Can you work these out from the model? Positions are in its coordinate system, mm. A direction names the side the tool comes from. Give positions to 0.01 mm unless a question says otherwise; leave off trailing zeros. Loops run counter-clockwise (first coordinate to the right, second up) from the corner with the lowest first, then second, coordinate; pieces in that order, holes last. Notation, with made-up numbers: M 85.5,53.5 L 108.5,53.5 A26 ccw 108.5,78.5 Z; hole C 88.5,56 d1. An arc over 180 degrees is marked long. Answer as a JSON object with one key per item and string values.
```python
from build123d import *

# Parameters (mm, degrees)
BOSS_EXTRUDE1_DEPTH = 60
SKETCH2_W           = 45
SKETCH2_H           = 21
CUT_EXTRUDE1_DEPTH  = 6
SKETCH3_W           = 6
SKETCH3_H           = 6
BOSS_EXTRUDE2_DEPTH = 18


with BuildPart() as part:
    # Sketch1 → Boss-Extrude1 (new body)
    with BuildSketch(Plane.XY):
        Polygon((50, 0), (-50, 0), (-69.206794991, 50), (-63.605822035, 52.151534787), (-45.877360691, 6), (45.877360691, 6), (63.605822035, 52.151534787), (69.206794991, 50), align=None)
    extrude(amount=BOSS_EXTRUDE1_DEPTH)

    # Sketch2 → Cut-Extrude1 (cut)
    with BuildSketch(Plane.XZ):
        with Locations((0, 18.669109879)):
            Rectangle(SKETCH2_W, SKETCH2_H)
    extrude(amount=-CUT_EXTRUDE1_DEPTH, mode=Mode.SUBTRACT)

    # Sketch3 → Boss-Extrude2 (add)
    with BuildSketch(Plane.XZ):
        with Locations((-19.5, 40.5)):
            Rectangle(SKETCH3_W, SKETCH3_H)
        with Locations((19.5, 40.5)):
            Rectangle(SKETCH3_W, SKETCH3_H)
    extrude(amount=BOSS_EXTRUDE2_DEPTH)


solid = part.part
```
1) For faces 1 (the flat face through (-16.5, -9, 40)), 2 (the flat face through (-20, -9, 43.5)), 3 (the flat face through (0, 3, 8.169)), 4 (the flat face through (-1, 6, 30)), which set-ups out of +Z, -Z, +X, -X, +Y, -Y let a thin tool reach every point of the face, with its end or its side?
Answer list:
{"face 1": "+Z, -Z, -Y", "face 2": "+Z, +X, -X, -Y", "face 3": "+Y, -Y", "face 4": "+Z, -Z, +Y"}
2) Suppose I cut it at D-D, the plane z = 54.5. Write out the boundary of the cut face in (x, y), and give its area (3 significant figures).
Answer list:
{"outline": "M -69.21,50 L -50,0 L 50,0 L 69.21,50 L 63.61,52.15 L 45.88,6 L -45.88,6 L -63.61,52.15 Z", "area": "1,190 mm^2"}
3) If we mould it in two halves opening along X, with no side actions, what happens to faces 5 (the flat face through (66.37, 51.09, 29.58)), 6 (the flat face through (0, 3, 29.169)), 7 (the flat face through (19, -9, 37.5))? For each: +X half, -X half, draft (parallel to the pull), parting line (faces both ways), or undercut.
Answer list:
{"face 5": "+X half", "face 6": "undercut", "face 7": "draft"}
4) Suppose I cut it at A-A, the plane x = 14. Write out the boundary of the cut face in (y, z), and give its area (3 significant figures).
Answer list:
{"outline": "M 0,0 L 6,0 L 6,8.17 L 0,8.17 Z; M 0,29.17 L 6,29.17 L 6,60 L 0,60 Z", "area": "234 mm^2"}
5) Suppose I cut it at B-B, the plane z = 24.5. Write out the boundary of the cut face in (x, y).
Answer list:
{"outline": "M -69.21,50 L -50,0 L -22.5,0 L -22.5,6 L -45.88,6 L -63.61,52.15 Z; M 22.5,0 L 50,0 L 69.21,50 L 63.61,52.15 L 45.88,6 L 22.5,6 Z"}
6) Will these pins go through, and if not, where does the flat tip stop? pin 1 Ø3 at (x, y) = (-6, 4) entering from -Z; pin 2 Ø6.5 at (x, y) = (-21, -5.5) entering from -Z; pin 3 Ø18 at (x, z) = (-6.5, 29.5) entering from -Y; pin 4 Ø6.5 at (y, z) = (-7, 41) entering from -X.
Answer list:
{"pin 1": "z = 0", "pin 2": "z = 37.5", "pin 3": "y = 0", "pin 4": "x = -22.5"}
7) Suppose I cut it at C-C, the plane y = 11.5. Write out the boundary of the cut face in (x, z).
Answer list:
{"outline": "M -54.42,0 L -47.99,0 L -47.99,60 L -54.42,60 Z; M 47.99,0 L 54.42,0 L 54.42,60 L 47.99,60 Z"}
8) Please list where these lines run through material, in increasing order: line 1 along Z through (x, y) = (1, 3.5); line 2 along Y through (x, z) = (-23.5, 41); line 3 along X through (y, z) = (43.5, 51.5). Write a range as from..to.
Answer list:
{"line 1": "0..8.17, 29.17..60", "line 2": "0..6", "line 3": "-66.71..-60.28, 60.28..66.71"}
